Geometry check sheet. Reference: the model listing, model coordinates, mm. Face numbers are marked on the shaded views. A direction names the side the tool comes from. Round coordinates to 2 decimals unless told otherwise and drop trailing zeros. Order: outer loops, then holes, each group sorted by start corner. A loop starts at its lowest first (then second) coordinate and runs counter-clockwise, first axis right, second up.
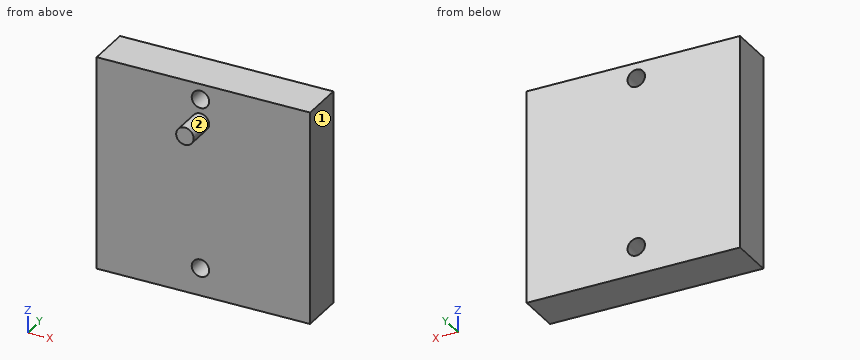
```python
from build123d import *

# Parameters (mm, degrees)
F0_W     = 93.267471
F0_H     = 93.26747
F1_DEPTH = 19.05
F2_R     = 3.814712
F3_DEPTH = 12.7
F5_D     = 7.62


with BuildPart() as f1:
    # F0 (on Front) → F1 (new body)
    with BuildSketch(Plane.XZ):
        with Locations((1.279228, 8.954607)):
            Rectangle(F0_W, F0_H)
    extrude(amount=F1_DEPTH)

    # F2 (on face) → F3 (join)
    with BuildSketch(Plane.XZ.offset(19.05)):
        with Locations((0, 38.842063)):
            Circle(F2_R)
    extrude(amount=F3_DEPTH)

    # F5 (through all)
    with Locations(Plane.XZ.offset(19.05)):
        with Locations((0, 48.843313), (0, -25.584593)):
            Hole(F5_D / 2)


solid = f1.part
```
(1) Depth check by flat-ended pin: P1, Ø3, axis at x = -35, z = -6.5, coming from the -Y side. Enter the tip coordinate at first touch or a pass-through.
Returned:
P1: stops at y = -19.05
(2) Sectioned sample at B-B, the plane z = 36.5. Record the cut outline in (x, y), and give its area (3 significant figures).
Returned:
outline: (-45.35, -19.05) - (-3.01, -19.05) - (-3.01, -31.75) - (3.01, -31.75) - (3.01, -19.05) - (47.91, -19.05) - (47.91, 0) - (-45.35, 0) - close
area: 1,850 mm2
(3) Sectioned sample at C-C, the plane x = 35. Record the cut outline in (y, z).
Returned:
outline: (-19.05, -37.68) - (0, -37.68) - (0, 55.59) - (-19.05, 55.59) - close
(4) Material ranges on line 1 (Z direction, x = 0, y = -5.25); line 2 (Y direction, x = -24.5, z = 12.5), recorded low to high.
Returned:
line 1: z = -37.68 to -29.39, -21.77 to 45.03, 52.65 to 55.59
line 2: y = -19.05 to 0
(5) Set-up check for the marked faces 1 and 2: record each of +Z, -Z, +X, -X, +Y, -Y from which the full face is reachable in a straight line by a thin tool's end or side.
Returned:
face 1: +Z, -Z, +X, +Y, -Y
face 2: -Y
(6) Sectioned sample at D-D, the plane y = -28. Record the cut outline in (x, z).
Returned:
outline: circle Ø7.63 at (0, 38.84)
(7) Sectioned sample at A-A, the plane x = 0. Record the cut outline in (y, z), and give its area (3 significant figures).
Returned:
outline: (-31.75, 35.03) - (-19.05, 35.03) - (-19.05, -21.77) - (0, -21.77) - (0, 45.03) - (-19.05, 45.03) - (-19.05, 42.66) - (-31.75, 42.66) - close; (-19.05, -37.68) - (0, -37.68) - (0, -29.39) - (-19.05, -29.39) - close; (-19.05, 52.65) - (0, 52.65) - (0, 55.59) - (-19.05, 55.59) - close
area: 1,580 mm2
